Check sheet for the drawn part. Datum: minimum x, y, z corner. Units: mm. A direction names the side the tool comes from. Coordinates: 2 decimals unless noted, no trailing zeros. Order: outer loops, then holes, each group sorted by start corner. A loop starts at its lowest first (then second) coordinate and runs counter-clockwise, first axis right, second up. Notation, with made-up numbers: M -14,-21 L 35,-21 A24 cw 35,-8 Z; hole C 67.25,-16 d3. An arc over 180 degrees is marked long. Return JSON: item names as keys, results as strings. Group by question number.
Q1. Access from +Z, -Z, +X, -X, +Y, -Y to the whole of each face (thin tool, end or side, straight path). Record for the marked faces 1 and 2.
Q2. Section check A-A, the plane y = 23.5. Enter the section's corners in (x, z), then the cut area to 3 significant figures.
Q3. Section check C-C, the plane z = 22.5. Enter the section's corners in (x, y), then the cut area to 3 significant figures.
Q4. Thickness scan on probe 1 along X at (y, z) = (24.25, 45.5); probe 2 along Z at (x, y) = (95.5, 18); probe 3 along X at (y, z) = (14, 6). Record the ranges inside material, lowest first.
Q5. Mould release check, pull along Z, two halves, no side actions. Record for the marked faces 3, 4 and 5: pulls with the +Z half, pulls with the -Z half, needs draft (parallel to the pull), parting line crosses it, or undercut.
Q6. Section check B-B, the plane x = 43.5. Enter the section's corners in (y, z), then the cut area to 3 significant figures.
Q7. Section check D-D, the plane x = 95.5. Enter the section's corners in (y, z), then the cut area to 3 significant figures.
Q8. Go/stop test with flat-tipped pins: pin 1 Ø3 at (x, z) = (20.5, 11.5) entering from +Y; pin 2 Ø6 at (x, z) = (62.5, 9) entering from -Y. Record where each tip stops, or that it passes through.
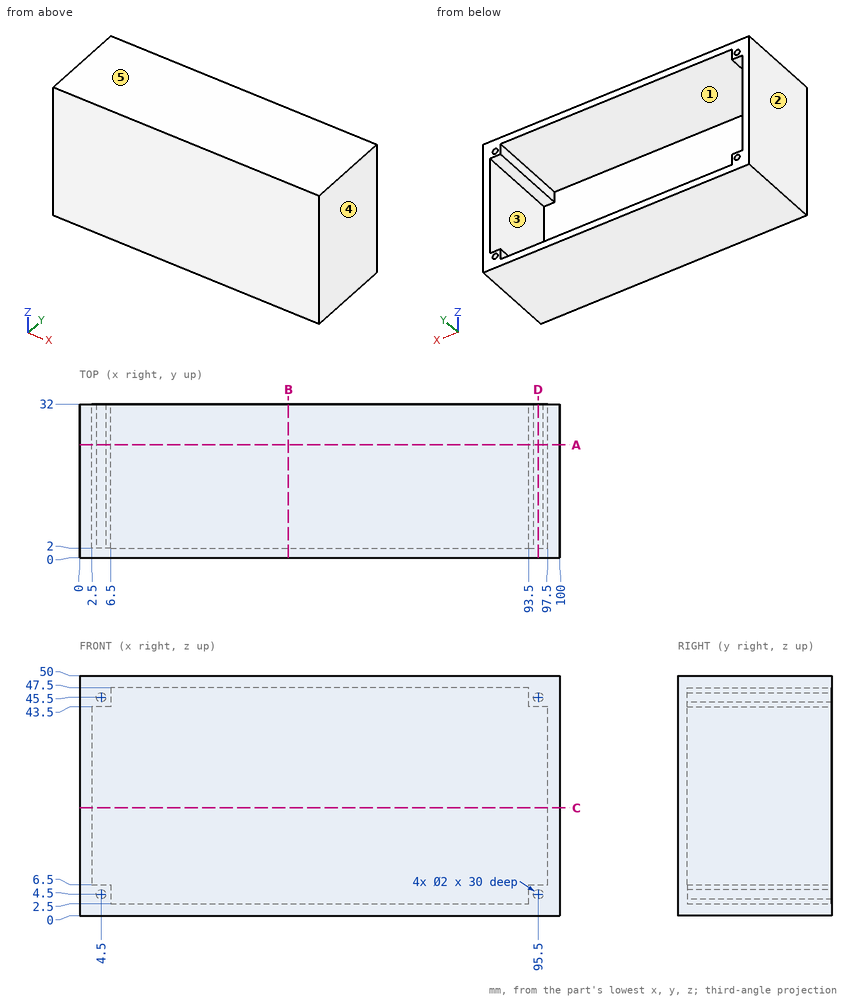
Numbers:
{
 "1": {"face 1": "+Y", "face 2": "+Z, -Z, -X, +Y, -Y"},
 "2": {"outline": "M 0,0 L 100,0 L 100,50 L 0,50 Z; hole M 2.5,6.5 L 6.5,6.5 L 6.5,2.5 L 93.5,2.5 L 93.5,6.5 L 97.5,6.5 L 97.5,43.5 L 93.5,43.5 L 93.5,47.5 L 6.5,47.5 L 6.5,43.5 L 2.5,43.5 Z; hole C 4.5,4.5 d2; hole C 4.5,45.5 d2; hole C 95.5,4.5 d2; hole C 95.5,45.5 d2", "area": "776 mm2"},
 "3": {"outline": "M 0,0 L 100,0 L 100,32 L 97.5,32 L 97.5,2 L 2.5,2 L 2.5,32 L 0,32 Z", "area": "350 mm2"},
 "4": {"probe 1": "x = 0 to 3.5, 5.5 to 6.5, 93.5 to 94.5, 96.5 to 100", "probe 2": "z = 0 to 3.5, 5.5 to 6.5, 43.5 to 44.5, 46.5 to 50", "probe 3": "x = 0 to 6.5, 93.5 to 100"},
 "5": {"face 3": "undercut", "face 4": "needs draft", "face 5": "pulls with the +Z half"},
 "6": {"outline": "M 0,0 L 32,0 L 32,2.5 L 2,2.5 L 2,47.5 L 32,47.5 L 32,50 L 0,50 Z", "area": "250 mm2"},
 "7": {"outline": "M 0,0 L 32,0 L 32,3.5 L 2,3.5 L 2,5.5 L 32,5.5 L 32,6.5 L 2,6.5 L 2,43.5 L 32,43.5 L 32,44.5 L 2,44.5 L 2,46.5 L 32,46.5 L 32,50 L 0,50 Z", "area": "370 mm2"},
 "8": {"pin 1": "stops at y = 2", "pin 2": "stops at y = 0"}
}
